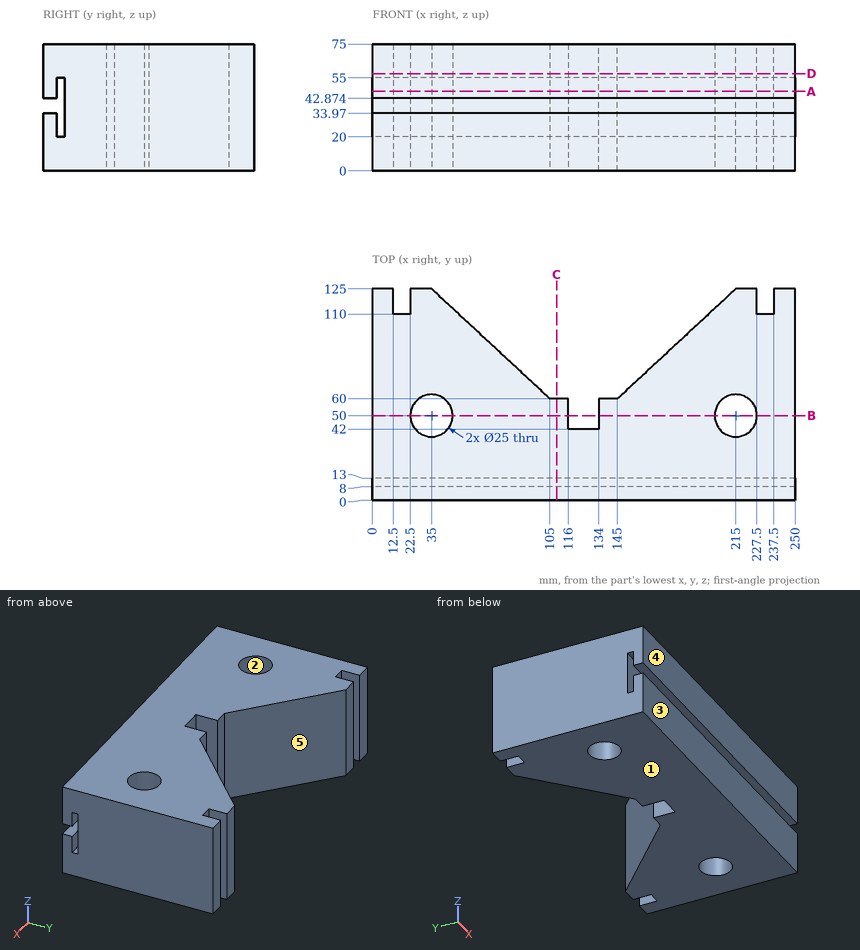
The figure shows three views and two pictorial views of one solid part (mm, origin at its lowest corner). Answer the questions. A direction names the side the tool comes from. Give positions to 0.01 mm unless a question says otherwise; leave off trailing zeros. Loops run counter-clockwise (first coordinate to the right, second up) from the corner with the lowest first, then second, coordinate; pieces in that order, holes last. Notation, with made-up numbers: M -2,-21 L 16,-21 A11 cw 16,-5 Z; hole C 86,-20 d6. An arc over 180 degrees is marked long. Write each question's results on one line, items separated by ' | '.
1. Section C-C on x = 109 is taken. Give the vertices of the cut face in (y, z).
Values:
outline: M 0,0 L 60,0 L 60,75 L 0,75 L 0,42.87 L 8,42.87 L 8,55 L 13,55 L 13,20 L 8,20 L 8,33.97 L 0,33.97 Z
2. Section A-A on z = 47 is taken. Give the vertices of the cut face in (x, y), plus the area to 3 significant figures.
Values:
outline: M 0,0 L 250,0 L 250,8 L 0,8 Z; M 0,13 L 250,13 L 250,125 L 237.5,125 L 237.5,110 L 227.5,110 L 227.5,125 L 215,125 L 145,60 L 134,60 L 134,42 L 116,42 L 116,60 L 105,60 L 35,125 L 22.5,125 L 22.5,110 L 12.5,110 L 12.5,125 L 0,125 Z; hole C 35,50 d25; hole C 215,50 d25 | area: 21,200 mm^2
3. Section B-B on y = 50 is taken. Give the vertices of the cut face in (x, z).
Values:
outline: M 0,0 L 22.5,0 L 22.5,75 L 0,75 Z; M 47.5,0 L 116,0 L 116,75 L 47.5,75 Z; M 134,0 L 202.5,0 L 202.5,75 L 134,75 Z; M 227.5,0 L 250,0 L 250,75 L 227.5,75 Z
4. Section D-D on z = 57.5 is taken. Give the vertices of the cut face in (x, y), plus the area to 3 significant figures.
Values:
outline: M 0,0 L 250,0 L 250,125 L 237.5,125 L 237.5,110 L 227.5,110 L 227.5,125 L 215,125 L 145,60 L 134,60 L 134,42 L 116,42 L 116,60 L 105,60 L 35,125 L 22.5,125 L 22.5,110 L 12.5,110 L 12.5,125 L 0,125 Z; hole C 35,50 d25; hole C 215,50 d25 | area: 22,500 mm^2
5. Given pin 1 (13.5 mm diameter, centred on x = 80.5, z = 50, fed in from +Y); pin 2 (20 mm diameter, centred on x = 35, y = 50, fed in from +Z); pin 3 (9 mm diameter, centred on x = 112, z = 49, fed in from +Y); pin 4 (5 mm diameter, centred on x = 233.5, z = 39.5, fed in from +Y), each flat-ended and moving along its own axis, determine where each tip first touches the part or whether it passes through.
Values:
pin 1: stops at y = 89.02 | pin 2: passes through | pin 3: stops at y = 60 | pin 4: stops at y = 110
6. Straight lines are drawn through the part: line 1 (Y direction, x = 35, z = 47); line 2 (Y direction, x = 215, z = 35); line 3 (Y direction, x = 33, z = 29.5). For each, find the intervals that lie inside material, in ascending order. Write a range as [from, to].
Values:
line 1: y = [0, 8], [13, 37.5], [62.5, 125] | line 2: y = [13, 37.5], [62.5, 125] | line 3: y = [0, 8], [13, 37.66], [62.34, 125]
7. The mould has two halves that part along Y. Classify the marked faces 1, 2 and 3: pulls with the +Y half, pulls with the -Y half, needs draft (parallel to the pull), parting line crosses it, or undercut.
Values:
face 1: needs draft | face 2: undercut | face 3: pulls with the -Y half
8. A tool of negligible diameter and unlimited length cuts with its end or side. For the marked faces 4 and 5, from which of +Z, -Z, +X, -X, +Y, -Y can it reach the whole face along a straight path? Write none if from no direction.
Values:
face 4: +Z, -Z, +X, -X, -Y | face 5: +Z, -Z, +Y
